Check sheet for the modelled part. Datum: model origin and axes. Units: mm. Face numbers are marked on the shaded views. A direction names the side the tool comes from. Coordinates: 2 decimals unless noted, no trailing zeros. Loops run counter-clockwise (first coordinate to the right, second up) from the corner with the lowest first, then second, coordinate; pieces in that order, holes last. Notation, with made-up numbers: M -24,-20.5 L -9,-20.5 A24 ccw -9,-6.5 Z; hole C -18,-36.75 d3. An arc over 180 degrees is marked long. Use CSV: the item, a comma, the result in double quotes. Start each with the question number.
(1) Section check B-B on x = 2.75. Record the cut outline in (y, z).
(2) Set-up check for the marked faces 1 and 2: record each of +Z, -Z, +X, -X, +Y, -Y from which the full face is reachable in a straight line by a thin tool's end or side.
(3) Scan lines: line 1 (Z direction, x = 8.5, y = 0); line 2 (Z direction, x = 3.5, y = 0); line 3 (Y direction, x = 7, z = -3.5). Record each from-to range of solid material in increasing order.
(4) Section check C-C on x = 11. Record the cut outline in (y, z), and give its area (3 significant figures).
(5) Go/stop test with flat-tipped pins: pin 1 Ø5 at (x, z) = (10, 0.5) entering from +Y; pin 2 Ø1.5 at (x, z) = (2.5, 7.5) entering from +Y; pin 3 Ø3 at (x, y) = (9, -2.5) entering from -Z. Record where each tip stops, or that it passes through.
(6) Section check A-A on y = 0. Record the cut outline in (x, z), and give its area (3 significant figures).
Autodesk Inventor part; units mm, degrees
ref_plane "Work Plane1" through (31.5112, 0, 0) normal (0, 0, 1) x (-1, 0, 0)
ref_plane "YZ Plane" through (0, 0, 0) normal (1, 0, 0) x (0, 1, 0)
ref_plane "XZ Plane" through (0, 0, 0) normal (0, 1, 0) x (-1, 0, 0)
sketch "Skizze1" plane through (0, 0, 0) normal (1, 0, 0) x (0, 1, 0)
  line L0 (5.4848, -9.5) -> (-5.4848, -9.5)
  line L1 (-5.4848, -9.5) -> (-10.9697, 0)
  line L2 (-10.9697, 0) -> (-5.4848, 9.5)
  line L3 (-5.4848, 9.5) -> (5.4848, 9.5)
  line L4 (5.4848, 9.5) -> (10.9697, 0)
  line L5 (10.9697, 0) -> (5.4848, -9.5)
  point P0 (0, 0)
  point P1 (0, 0)
  dimension "d0" = 21.9393
extrude "Körper" add sketch "Skizze1" along normal blind 8
sketch "Skizze2" plane through (8, 0, 0) normal (1, 0, 0) x (0, 0, -1)
  circle A0 centre (0, 0) radius 8.7
  dimension "d7" = 17.4
extrude "Ring" add sketch "Skizze2" along normal blind 4
sketch "Skizze3" plane through (0, 0, 0) normal (0, 0, 1) x (1, 0, 0)
  line L0 (0, 5.4848) -> (0, 10.9697)
  line L1 (0, 10.9697) -> (8, 10.9697)
  line L2 (8, 5.4848) -> (8, 10.9697)
  line L3 (-1.6, 0) -> (9.6, 0)
  line L4 (0, 8.7) -> (1.3104, 10.9697)
  line L5 (6.6896, 10.9697) -> (8, 8.7)
  dimension "d3" = 30
  dimension "d4" = 30
  dimension "d5" = 17.4
  dimension "d6" = 17.4
revolve "Fase1" cut sketch "Skizze3" angle 360 about axis through (-10, 0, 0) along (1, 0, 0)
sketch "Skizze4" plane through (0, 0, 0) normal (-1, 0, 0) x (0, 0, 1)
  line L0 (0, -15.3575) -> (0, 15.3575)
  line L1 (-13.3, 0) -> (13.3, 0)
  point P0 (0, 0)
hole "Gewinde" at (0, 0, 0) direction (1, 0, 0) diameter 10.106 end through all
chamfer "Fase2" distance 0.9472 angle 30 1 edges at (0, 0, -5.053) measured on face at (0, 7.3878, -0.897)
chamfer "Fase3" distance 0.9472 angle 30 1 edges at (12, 0, -5.053) measured on face at (12, -1.0971, -7.3511)
ref_plane "Work Plane1" through (31.5112, 0, 0) normal (0, 0, 1) x (-1, 0, 0)
equation "\"d0\" = 1.1547 * SW"
equation "\"d1\" = KOH1"
equation "\"d7\" = SD2"
equation "\"d8\" = KOH - KOH1"
equation "\"d3\" = ANG1"
equation "\"d4\" = ANG2"
equation "\"d5\" = SW0"
equation "\"d6\" = SW01"
equation "\"d10\" = -0.5 * GD1 + 0.5 * NND"
equation "\"d46\" = -0.5 * GD1 + 0.5 * NND"
equation "\"d12\" = -0.5 * GD1 + 0.5 * NND"
equation "\"d47\" = -0.5 * GD1 + 0.5 * NND"
equation "\"ANG1\" = 30deg"
equation "\"ANG2\" = 30deg"
equation "\"NND\" = 12"
equation "\"KOH1\" = 8"
equation "\"KOH\" = 12"
equation "\"SW\" = 19"
equation "\"SW0\" = 17.4"
equation "\"SW01\" = SW0"
equation "\"SD2\" = SW0"
equation "\"GUL\" = 0.541266 * PTC"
equation "\"THREADDIA\" = 12"
equation "\"TOA\" = 30deg"
equation "\"PTC\" = 1.75"
equation "\"GAL\" = 0.541266 * PTC"
equation "\"E0\" = 1.155 * SW"
properties part number "DIN 985 - M12" material "Steel, Mild"
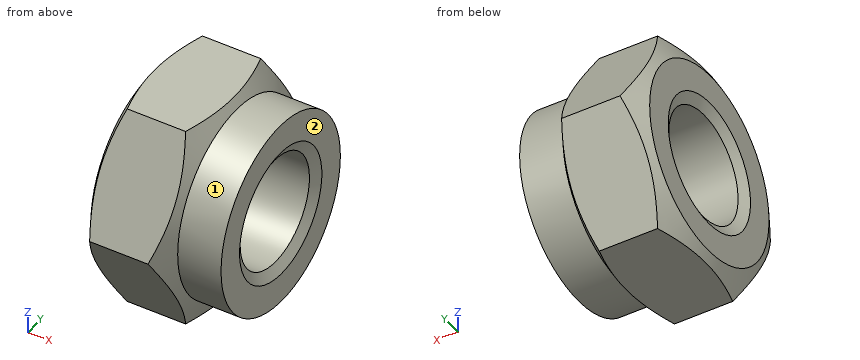
Outcome:
1,outline,"M -10.97,0 L -5.48,-9.5 L 5.48,-9.5 L 10.97,0 L 5.48,9.5 L -5.48,9.5 Z; hole C 0,0 d10.11"
2,face 1,"+X"
2,face 2,"+Z, -Z, +X, +Y, -Y"
3,line 1,"z = -8.7 to -5.05, 5.05 to 8.7"
3,line 2,"z = -9.5 to -5.05, 5.05 to 9.5"
3,line 3,"y = -8.95 to -3.64, 3.64 to 8.95"
4,outline,"C 0,0 d17.4; hole C 0,0 d10.11"
4,area,"158 mm²"
5,pin 1,"stops at y = 9.55"
5,pin 2,"stops at y = 7.07"
5,pin 3,"stops at z = -9.26"
6,outline,"M 0,-8.7 L 0.46,-9.5 L 7.54,-9.5 L 8,-8.7 L 12,-8.7 L 12,-6 L 11.45,-5.05 L 0.55,-5.05 L 0,-6 Z; M 0,6 L 0.55,5.05 L 11.45,5.05 L 12,6 L 12,8.7 L 8,8.7 L 7.54,9.5 L 0.46,9.5 L 0,8.7 Z"
6,area,"98.6 mm²"
